from build123d import *

# Parameters (mm, degrees)
EXTRUDE_1_DEPTH        = 20
SKETCH_2_R             = 1.4
CUT_EXTRUDE_1_DEPTH    = 40
SKETCH_1_3_W           = 110
SKETCH_1_3_H           = 2
EXTRUDE_2_DEPTH        = 10
EXTRUDE_3_DEPTH        = 120
CUT_EXTRUDE_2_DEPTH    = 20
SKETCH_5_W             = 25
SKETCH_5_H             = 5.4
CUT_EXTRUDE_3_DEPTH    = 2.5
PATTERN_LINEAR_1_COUNT = 11
PATTERN_LINEAR_1_PITCH = 10
CHAMFER_1_SIZE         = 3
SKETCH_6_R             = 2.9
CUT_EXTRUDE_4_DEPTH    = 2
CHAMFER_2_SIZE         = 1.6
CHAMFER_2_SIZE_2       = 2
CHAMFER_3_SIZE         = 2.5
CHAMFER_4_SIZE         = 5


with BuildPart() as part:
    # 스케치1 → 보스-돌출1 (new, symmetric)
    with BuildSketch(Plane(origin=(0, 0, 0), x_dir=(0, 0, -1), z_dir=(1, 0, 0))):
        Polygon((-10, 29.1), (-10, 27.1), (-10, 0), (0, 0), (0, 29.1), align=None)
    extrude(amount=EXTRUDE_1_DEPTH, both=True)

    # 스케치2 → 컷-돌출1 (cut)
    with BuildSketch(Plane.XY):
        with Locations((17, 3)):
            Circle(SKETCH_2_R)
        with Locations((17, 17)):
            Circle(SKETCH_2_R)
        with Locations(Location((-17, 3, 0), (0, 0, 180))):
            Circle(SKETCH_2_R)
        with Locations(Location((-17, 17, 0), (0, 0, 180))):
            Circle(SKETCH_2_R)
    extrude(amount=CUT_EXTRUDE_1_DEPTH, mode=Mode.SUBTRACT)

    # 스케치1<3> → 보스-돌출2 (add, symmetric)
    with BuildSketch(Plane(origin=(0, 0, 0), x_dir=(0, 0, -1), z_dir=(1, 0, 0))):
        with Locations((-65, 28.1)):
            Rectangle(SKETCH_1_3_W, SKETCH_1_3_H)
    extrude(amount=EXTRUDE_2_DEPTH, both=True)

    # 스케치3 → 보스-돌출3 (add)
    with BuildSketch(Plane.XY):
        Polygon((7.5, 29.1), (-7.5, 29.1), (-7.5, 31.6), (-10.4, 34.6), (-10.4, 34.7), (-8.25, 37.2), (8.25, 37.2), (10.4, 34.7), (10.4, 34.6), (7.5, 31.6), align=None)
    extrude(amount=EXTRUDE_3_DEPTH)

    # 스케치4 → 컷-돌출2 (cut)
    with BuildSketch(Plane(origin=(0, 37.2, 0), x_dir=(1, 0, 0), z_dir=(0, 1, 0))):
        with BuildLine():
            Line((-3.343759528, -13.296813629), (3.343759528, -13.296813629))
            ThreePointArc((3.343759528, -13.296813629), (6.943759528, -16.896813629), (3.343759528, -20.496813629))
            Line((3.343759528, -20.496813629), (-3.343759528, -20.496813629))
            ThreePointArc((-3.343759528, -20.496813629), (-6.943759528, -16.896813629), (-3.343759528, -13.296813629))
        make_face()
    extrude(amount=-CUT_EXTRUDE_2_DEPTH, mode=Mode.SUBTRACT)

    # 스케치5 → 컷-돌출3 (cut)
    with BuildSketch(Plane(origin=(0, 37.2, 0), x_dir=(1, 0, 0), z_dir=(0, 1, 0))):
        with Locations((0, -10)):
            Rectangle(SKETCH_5_W, SKETCH_5_H)
    cut_extrude_3 = extrude(amount=-CUT_EXTRUDE_3_DEPTH, mode=Mode.SUBTRACT)

    # 선형 패턴1: 컷-돌출3 ×11
    with Locations(*[(0, 0, i * PATTERN_LINEAR_1_PITCH) for i in range(1, PATTERN_LINEAR_1_COUNT)]):
        add(cut_extrude_3, mode=Mode.SUBTRACT)

    # 모따기1
    chamfer_1_edges = [part.edges().sort_by_distance(p)[0] for p in [
        (0, 27.1, 10),
    ]]
    chamfer(chamfer_1_edges, length=CHAMFER_1_SIZE)

    # 스케치6 → 컷-돌출4 (cut)
    with BuildSketch(Plane(origin=(0, 0, 0), x_dir=(-1, 0, 0), z_dir=(0, 0, -1))):
        with Locations((-17, 3)):
            Circle(SKETCH_6_R)
        with Locations((-17, 17)):
            Circle(SKETCH_6_R)
        with Locations((17, 17)):
            Circle(SKETCH_6_R)
        with Locations((17, 3)):
            Circle(SKETCH_6_R)
    extrude(amount=-CUT_EXTRUDE_4_DEPTH, mode=Mode.SUBTRACT)

    # 모따기2
    # the kernel refuses this chamfer: 2, 1.6 mm, written as the material it adds along each edge
    with BuildSketch(Plane(origin=(17, 3, 2), x_dir=(-1, 0, 0), z_dir=(0, -1, 0))) as chamfer_2_piece_1_section:
        Polygon((2.9 - CHAMFER_2_SIZE, 0), (2.9, CHAMFER_2_SIZE_2), (2.9, 0), align=None)
    chamfer_2_piece_1 = revolve(axis=Axis((17, 3, 2), (0, 0, -1)), mode=Mode.PRIVATE)
    chamfer_2_piece_1 = chamfer_2_piece_1 - Plane(origin=(17, 3, 0.956092246), x_dir=(1, 0, 0), z_dir=(0, 0, -1)) * Cylinder(1.4, 12, mode=Mode.PRIVATE)
    chamfer_2_piece_1 = split(chamfer_2_piece_1, bisect_by=Plane(origin=(19.173240308, 3, 0), z_dir=(0, 0, 1)), keep=Keep.TOP, mode=Mode.PRIVATE)
    add(chamfer_2_piece_1)
    with BuildSketch(Plane(origin=(-17, 3, 2), x_dir=(-1, 0, 0), z_dir=(0, -1, 0))) as chamfer_2_piece_2_section:
        Polygon((2.9 - CHAMFER_2_SIZE, 0), (2.9, CHAMFER_2_SIZE_2), (2.9, 0), align=None)
    chamfer_2_piece_2 = revolve(axis=Axis((-17, 3, 2), (0, 0, -1)), mode=Mode.PRIVATE)
    chamfer_2_piece_2 = chamfer_2_piece_2 - Plane(origin=(-17, 3, 0.956092246), x_dir=(-1, 0, 0), z_dir=(0, 0, -1)) * Cylinder(1.4, 12, mode=Mode.PRIVATE)
    chamfer_2_piece_2 = split(chamfer_2_piece_2, bisect_by=Plane(origin=(-14.826759692, 3, 0), z_dir=(0, 0, 1)), keep=Keep.TOP, mode=Mode.PRIVATE)
    add(chamfer_2_piece_2)
    with BuildSketch(Plane(origin=(-17, 17, 2), x_dir=(-1, 0, 0), z_dir=(0, -1, 0))) as chamfer_2_piece_3_section:
        Polygon((2.9 - CHAMFER_2_SIZE, 0), (2.9, CHAMFER_2_SIZE_2), (2.9, 0), align=None)
    chamfer_2_piece_3 = revolve(axis=Axis((-17, 17, 2), (0, 0, -1)), mode=Mode.PRIVATE)
    chamfer_2_piece_3 = chamfer_2_piece_3 - Plane(origin=(-17, 17, 0.956092246), x_dir=(-1, 0, 0), z_dir=(0, 0, -1)) * Cylinder(1.4, 12, mode=Mode.PRIVATE)
    chamfer_2_piece_3 = split(chamfer_2_piece_3, bisect_by=Plane(origin=(-14.826759692, 17, 0), z_dir=(0, 0, 1)), keep=Keep.TOP, mode=Mode.PRIVATE)
    add(chamfer_2_piece_3)
    with BuildSketch(Plane(origin=(17, 17, 2), x_dir=(-1, 0, 0), z_dir=(0, -1, 0))) as chamfer_2_piece_4_section:
        Polygon((2.9 - CHAMFER_2_SIZE, 0), (2.9, CHAMFER_2_SIZE_2), (2.9, 0), align=None)
    chamfer_2_piece_4 = revolve(axis=Axis((17, 17, 2), (0, 0, -1)), mode=Mode.PRIVATE)
    chamfer_2_piece_4 = chamfer_2_piece_4 - Plane(origin=(17, 17, 0.956092246), x_dir=(1, 0, 0), z_dir=(0, 0, -1)) * Cylinder(1.4, 12, mode=Mode.PRIVATE)
    chamfer_2_piece_4 = split(chamfer_2_piece_4, bisect_by=Plane(origin=(19.173240308, 17, 0), z_dir=(0, 0, 1)), keep=Keep.TOP, mode=Mode.PRIVATE)
    add(chamfer_2_piece_4)

    # 모따기3
    chamfer_3_edges = [part.edges().sort_by_distance(p)[0] for p in [
        (0, 37.2, 120),
        (0, 37.2, 0),
    ]]
    chamfer(chamfer_3_edges, length=CHAMFER_3_SIZE)

    # 모따기4
    chamfer_4_edges = [part.edges().sort_by_distance(p)[0] for p in [
        (-13.75, 29.1, 0),
        (-20, 29.1, 5),
        (20, 29.1, 5),
        (13.75, 29.1, 0),
    ]]
    chamfer(chamfer_4_edges, length=CHAMFER_4_SIZE)


solid = part.part
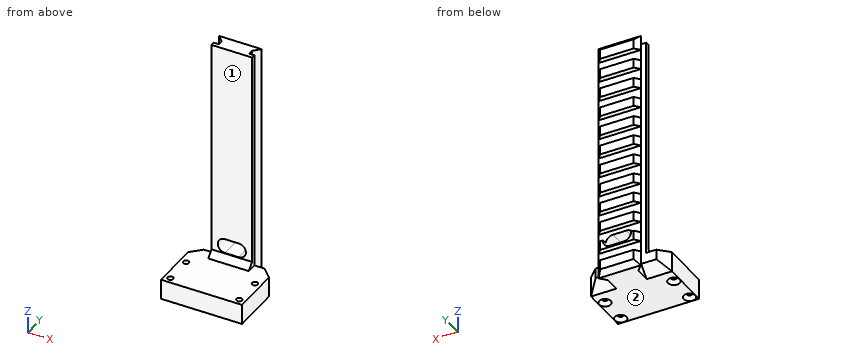
Here's how the part is built. I have some questions about the finished solid (model axes, mm). Face numbers are marked on the shaded views. A direction names the side the tool comes from. Coordinates: 2 decimals unless noted, no trailing zeros. Order: outer loops, then holes, each group sorted by start corner. A loop starts at its lowest first (then second) coordinate and runs counter-clockwise, first axis right, second up. Notation, with made-up numbers: (8, 73.25) -> (30, 73.25) arc R29 ccw to (30, 97.25) -> close; hole circle Ø9 at (-26.5, 3). An arc over 180 degrees is marked (long way). Answer in a Markdown table with one row per item.
(1) Please list where these lines run through material, in increasing order: probe 1 along Y at (x, z) = (17, 7); probe 2 along X at (y, z) = (3, 5.5); probe 3 along Y at (x, z) = (16, 9).
Answer key:
| item | result |
|---|---|
| probe 1 | 0 to 1.6, 4.4 to 15.6, 18.4 to 27.1 |
| probe 2 | -20 to -18.4, -15.6 to 15.6, 18.4 to 20 |
| probe 3 | 0 to 2.02, 3.98 to 16.02, 17.98 to 28.1 |
(2) On a 3-axis mill with a long thin cutter (end or side, diameter ignored), from which of +Z, -Z, +X, -X, +Y, -Y can I reach the whole of each face in a straight line? I mean the marked faces 1 and 2. Say none if no direction works.
Answer key:
| item | result |
|---|---|
| face 1 | +Z, +X, -X, -Y |
| face 2 | -Z, +X, -X, +Y, -Y |
(3) I want a section at C-C on z = 90.5. List the corners of the cut face in (x, y) for me.
Answer key:
| item | result |
|---|---|
| outline | (-10.4, 34.6) -> (-7.5, 31.6) -> (-7.5, 29.1) -> (-10, 29.1) -> (-10, 27.1) -> (10, 27.1) -> (10, 29.1) -> (7.5, 29.1) -> (7.5, 31.6) -> (10.4, 34.6) -> (10.4, 34.7) -> (-10.4, 34.7) -> close |
(4) Will these pins go through, and if not, where does the flat tip stop? pin 1 Ø4 at (x, z) = (-9.5, 73) entering from +Y; pin 2 Ø2.5 at (x, z) = (3.5, 30) entering from +Y; pin 3 Ø2 at (x, y) = (2.5, 36.5) entering from +Z; pin 4 Ø6 at (y, z) = (30, 89) entering from -X.
Answer key:
| item | result |
|---|---|
| pin 1 | y = 37.2 |
| pin 2 | y = 34.7 |
| pin 3 | z = 119.2 |
| pin 4 | x = -10 |
(5) I want a section at A-A on y = 3. List the corners of the cut face in (x, z) for me (3 decimals), then the cut area to 3 significant figures.
Answer key:
| item | result |
|---|---|
| outline | (-20, 0) -> (-19.9, 0) -> (-18.4, 1.875) -> (-18.4, 10) -> (-20, 10) -> close; (-15.6, 1.875) -> (-14.1, 0) -> (14.1, 0) -> (15.6, 1.875) -> (15.6, 10) -> (-15.6, 10) -> close; (18.4, 1.875) -> (19.9, 0) -> (20, 0) -> (20, 10) -> (18.4, 10) -> close |
| area | 338 mm^2 |
(6) I want a section at D-D on x = 11.5. List the corners of the cut face in (y, z) for me, then the cut area to 4 significant figures.
Answer key:
| item | result |
|---|---|
| outline | (0, 0) -> (24.1, 0) -> (29.1, 5) -> (29.1, 10) -> (0, 10) -> close |
| area | 278.5 mm^2 |
(7) I want a section at B-B on x = -17. List the corners of the cut face in (y, z) for me (3 decimals).
Answer key:
| item | result |
|---|---|
| outline | (0, 0) -> (0.1, 0) -> (1.6, 1.875) -> (1.6, 10) -> (0, 10) -> close; (4.4, 1.875) -> (5.9, 0) -> (14.1, 0) -> (15.6, 1.875) -> (15.6, 10) -> (4.4, 10) -> close; (18.4, 1.875) -> (19.9, 0) -> (24.1, 0) -> (27.1, 3) -> (27.1, 10) -> (18.4, 10) -> close |
